```python
from build123d import *

# Parameters (mm, degrees)
F0_W     = 24.13
F0_H     = 24.13
F1_DEPTH = 24.13
F3_D     = 2.3749
F3_DEPTH = 14.2875
F3_TIP   = 0.7134919421
F5_D     = 2.3749
F5_DEPTH = 14.3002
F5_TIP   = 0.7134919421
F7_D     = 2.3749
F7_DEPTH = 14.3002
F7_TIP   = 0.7134919421


with BuildPart() as f1:
    # F0 (on Top) → F1 (new body)
    with BuildSketch(Plane.XY):
        Rectangle(F0_W, F0_H)
    extrude(amount=F1_DEPTH)

    # F3
    with Locations(Plane.YZ.offset(12.065)):
        with Locations((0, 12.065)):
            Hole(F3_D / 2, depth=F3_DEPTH)
            with Locations((0, 0, -(F3_DEPTH + F3_TIP / 2))):  # 118° drill point
                Cone(0, F3_D / 2, F3_TIP, mode=Mode.SUBTRACT)

    # F5
    with Locations(Plane(origin=(0, 0, 0), x_dir=(1, 0, 0), z_dir=(0, 0, -1))):
        with Locations((0.0603985645, 0)):
            Hole(F5_D / 2, depth=F5_DEPTH)
            with Locations((0, 0, -(F5_DEPTH + F5_TIP / 2))):  # 118° drill point
                Cone(0, F5_D / 2, F5_TIP, mode=Mode.SUBTRACT)

    # F7
    with Locations(Plane(origin=(0, 12.065, 0), x_dir=(-1, 0, 0), z_dir=(0, 1, 0))):
        with Locations((0, 12.065)):
            Hole(F7_D / 2, depth=F7_DEPTH)
            with Locations((0, 0, -(F7_DEPTH + F7_TIP / 2))):  # 118° drill point
                Cone(0, F7_D / 2, F7_TIP, mode=Mode.SUBTRACT)


solid = f1.part
```
Can you work these out from the model? Positions are in its coordinate system, mm. A direction names the side the tool comes from. Coordinates: 2 decimals unless noted, no trailing zeros. Answer as CSV lines item,"result". Start each with the question number.
1) Thinking about a two-plate mould opening in Y: for faces 1 (the cylindrical face through (-1.683, 0.875, 12.868)), 2 (the flat face through (0, 0, 24.13)), 3 (the flat face through (0, -12.065, 12)), which applies, pulls with the +Y half, pulls with the -Y half, needs draft (parallel to the pull), parting line crosses it, or undercut?
2) I need wall thicknesses on line 1 (Z direction, x = 0, y = 4.25); line 2 (Y direction, x = 0.25, z = 1.75) (3 decimals). Which ranges of each line are inside material? Lowest first, please. Write a range as from..to.
3) For pin 1 (1.4 mm diameter, centred on y = 0, z = 12.065, fed in from +X), with a flat end and sliding along its axis, tell me the tip position at first contact or that it passes through.
4) Which directions (+Z, -Z, +X, -X, +Y, -Y) give clear straight access to the entire face, cutting with the end or side of a thin tool? Please do faces 4 (the cylindrical face through (0.94, -0.8, 5.71)), 5 (the flat face through (-12.065, 0, 12)), 6 (the cylindrical face through (6.389, 0.155, 13.242)), 7 (the cylindrical face through (-0.155, 6.358, 13.242)).
Check result:
1,face 1,"undercut"
1,face 2,"needs draft"
1,face 3,"pulls with the -Y half"
2,line 1,"z = 0..10.88, 13.25..24.13"
2,line 2,"y = -12.065..-1.172, 1.172..12.065"
3,pin 1,"stops at x = -2.52"
4,face 4,"-Z"
4,face 5,"+Z, -Z, -X, +Y, -Y"
4,face 6,"+X"
4,face 7,"+Y"
